Here's how the part is built. I have some questions about the finished solid (model axes, mm). A direction names the side the tool comes from. Give positions to 0.01 mm unless a question says otherwise; leave off trailing zeros. Loops run counter-clockwise (first coordinate to the right, second up) from the corner with the lowest first, then second, coordinate; pieces in that order, holes last. Notation, with made-up numbers: (73.25, 6) - (127.25, 6) arc R28 ccw to (127.25, 40) - close; hole circle Ø8 at (4, -4.5). An arc over 180 degrees is marked (long way). Return JSON: item names as keys, results as strings. Group by question number.
(1) For P1, Ø5, axis at y = 16, z = 29, coming from the +X side; P2, Ø8, axis at x = -4.5, y = 14.5, coming from the +Z side; P3, Ø10, axis at y = 6.5, z = 89.5, coming from the +X side, each with a flat end and sliding along its axis, tell me the tip position at first contact or that it passes through.
(2) If we section it at D-D (x = -33.5): Please give me the cut outline in (y, z), then the cut area to 3 significant figures.
(3) On a 3-axis mill with a long thin cutter (end or side, diameter ignored), from which of +Z, -Z, +X, -X, +Y, -Y can I reach the whole of each face in a straight line? I mean faces 1 (the flat face through (6.18, 25.04, 23.15)), 2 (the flat face through (-25.925, 25.044, 111.626)), 3 (the flat face through (55.765, 25.044, 116.994)), 4 (the flat face through (-100.978, 25.044, 52.985)). Say none if no direction works.
(4) If we mould it in two halves opening along X, with no side actions, what happens to faces 5 (the flat face through (36.461, 25.044, 32.903)), 6 (the flat face through (-66.89, 25.04, 19.25)), 7 (the flat face through (-25, 0, 56))? For each: released by +X, released by -X, zero draft, split by the parting line, or undercut.
(5) If we section it at C-C (y = 7): Please give me the cut outline in (x, z).
(6) I need wall thicknesses on probe 1 along X at (y, z) = (26.5, 41); probe 2 along Z at (x, y) = (52, 19.5); probe 3 along X at (y, z) = (34, 112.5). Which ranges of each line are inside material? Lowest first, please. Write a range as [from, to].
(7) If we section it at B-B (x = 42.5): Please give me the cut outline in (y, z), then the cut area to 3 significant figures.
(8) If we section it at A-A (z = 121.5): Please give me the cut outline in (x, y).
```python
from build123d import *

# Parameters (mm, degrees)
F1_DEPTH = 50.8


with BuildPart() as f1:
    # F0 (on Front) → F1 (new body)
    with BuildSketch(Plane.XZ):
        Polygon((-131.935537, 37.967242), (0, 0), (12.539328, 46.962254), (61.061069, 18.444592), (28.349791, 92.415459), (83.958983, 142.270118), (-8.723013, 96.433535), (-43.615054, 127.250195), (-70.87446, 67.588188), align=None)
    extrude(amount=-F1_DEPTH)


solid = f1.part
```
Values:
{
 "1": {"P1": "x = 57.5", "P2": "z = 100.5", "P3": "x = 31.85"},
 "2": {"outline": "(0, 9.64) - (50.8, 9.64) - (50.8, 118.32) - (0, 118.32) - close", "area": "5,520 mm2"},
 "3": {"face 1": "-Z, +Y, -Y", "face 2": "+Z, +Y, -Y", "face 3": "+X, +Y, -Y", "face 4": "+Z, -X, +Y, -Y"},
 "4": {"face 5": "undercut", "face 6": "released by -X", "face 7": "zero draft"},
 "5": {"outline": "(-131.94, 37.97) - (0, 0) - (12.54, 46.96) - (61.06, 18.44) - (28.35, 92.42) - (83.96, 142.27) - (-8.72, 96.43) - (-43.62, 127.25) - (-70.87, 67.59) - close"},
 "6": {"probe 1": "[-125.68, 10.95], [22.68, 51.09]", "probe 2": "[23.77, 38.93], [113.62, 126.46]", "probe 3": "[-50.35, -26.91], [23.76, 50.75]"},
 "7": {"outline": "(0, 29.35) - (50.8, 29.35) - (50.8, 60.42) - (0, 60.42) - close; (0, 105.1) - (50.8, 105.1) - (50.8, 121.77) - (0, 121.77) - close", "area": "2,420 mm2"},
 "8": {"outline": "(-46.24, 0) - (-37.1, 0) - (-37.1, 50.8) - (-46.24, 50.8) - close; (41.96, 0) - (60.79, 0) - (60.79, 50.8) - (41.96, 50.8) - close"}
}
